from build123d import *

# Parameters (mm, degrees)
F0_W     = 66
F0_H     = 26
F1_DEPTH = 1.6
F3_R     = 1.3
F4_DEPTH = 1.6


with BuildPart() as f1:
    # F0 (on Top) → F1 (new body)
    with BuildSketch(Plane.XY):
        with Locations((33, 13)):
            Rectangle(F0_W, F0_H)
    extrude(amount=F1_DEPTH)

    # F3 (on face) → F4 (cut, through all)
    with BuildSketch(Plane.XY.offset(1.6)):
        with BuildLine():
            Line((14.0246950766, 5.5), (11.9753049234, 5.5))
            ThreePointArc((11.9753049234, 5.5), (13, 5), (14.0246950766, 5.5))
        make_face()
        with BuildLine():
            ThreePointArc((14.0246950766, 5.5), (14.2292484695, 5.8769773053), (14.3, 6.3))
            ThreePointArc((14.3, 6.3), (12.5769773053, 7.5292484695), (11.9753049234, 5.5))
            Line((11.9753049234, 5.5), (14.0246950766, 5.5))
        make_face()
        with Locations((43.2, 12)):
            Circle(F3_R)
    extrude(amount=-F4_DEPTH, mode=Mode.SUBTRACT)


solid = f1.part
Could you check a few things on this model? Use its own coordinates, in mm. Give positions to 0.01 mm unless a question says otherwise; leave off trailing zeros. Write each loop counter-clockwise with the first axis right and the second up, starting at its lowest first coordinate (ties: lowest second). Pieces come first, ordered by that corner, then holes. Notation, with made-up numbers: (72, 57) -> (124, 57) arc R22 ccw to (124, 82) -> close; hole circle Ø6 at (76, 78.25). An arc over 180 degrees is marked (long way). Answer as a JSON object with one key per item and string values.
Q1. Suppose I cut it at A-A on y = 12. Write out the boundary of the cut face in (x, z), then the cut area to 3 significant figures.
Taken from the geometry:
{"outline": "(0, 0) -> (41.9, 0) -> (41.9, 1.6) -> (0, 1.6) -> close; (44.5, 0) -> (66, 0) -> (66, 1.6) -> (44.5, 1.6) -> close", "area": "101 mm²"}
Q2. Suppose I cut it at B-B on x = 43.2. Write out the boundary of the cut face in (y, z).
Taken from the geometry:
{"outline": "(0, 0) -> (10.7, 0) -> (10.7, 1.6) -> (0, 1.6) -> close; (13.3, 0) -> (26, 0) -> (26, 1.6) -> (13.3, 1.6) -> close"}
Q3. Please list where these lines run through material, in increasing order: L1, parallel to Y at x = 13, z = 0.6; L2, parallel to X at y = 6.3, z = 0.9; L3, parallel to Y at x = 43.2, z = 1.15.
Taken from the geometry:
{"L1": "y = 0 to 5, 7.6 to 26", "L2": "x = 0 to 11.7, 14.3 to 66", "L3": "y = 0 to 10.7, 13.3 to 26"}
Q4. We'd pull the mould along X, two halves only. Please class faces 1 (the flat face through (0, 13, 1)), 2 (the flat face through (33, 13, 0)), 3 (the cylindrical face through (44.44, 12.39, 0.81)): released by +X, released by -X, zero draft, split by the parting line, or undercut.
Taken from the geometry:
{"face 1": "released by -X", "face 2": "zero draft", "face 3": "undercut"}
Q5. Will this pin go through, and if not, where does the flat tip stop? pin 1 Ø3 at (x, y) = (13, 6.3) entering from +Z.
Taken from the geometry:
{"pin 1": "stops at z = 1.6"}
